Read the model definition and answer for the solid it produces. Units are mm, in the model's axes. Round coordinates to 2 decimals unless told otherwise and drop trailing zeros. Write each loop counter-clockwise with the first axis right and the second up, starting at its lowest first coordinate (ties: lowest second). Pieces come first, ordered by that corner, then holes. Notation, with made-up numbers: M 22.5,-20.5 L 53.5,-20.5 A23 ccw 53.5,4.5 Z; hole C 2.25,24 d7. An arc over 180 degrees is marked long. Use one line per item in the form item = value. Start each with the question number.
```python
from build123d import *

# Parameters (mm, degrees)
SKETCH_W  = 36
SKETCH_H  = 25
SKETCH_R  = 2
PAD_DEPTH = 11
FILLET_R  = 3


with BuildPart() as part:
    # Sketch → Pad (new body)
    with BuildSketch(Plane.XY):
        with Locations((0, 12.5)):
            Rectangle(SKETCH_W, SKETCH_H)
        with Locations((10, 16)):
            Circle(SKETCH_R, mode=Mode.SUBTRACT)
        with Locations((-10, 16)):
            Circle(SKETCH_R, mode=Mode.SUBTRACT)
    extrude(amount=PAD_DEPTH)

    # Fillet
    fillet_edges = [part.edges().sort_by_distance(p)[0] for p in [
        (-18, 25, 5.5),
        (18, 25, 5.5),
    ]]
    fillet(fillet_edges, radius=FILLET_R)


solid = part.part
```
Q1. Find section A-A on y = 16. Write down the section's boundary in (x, z).
Q2. For a pull along X with two mould halves and no side action, classify faces 1 (the face through (18, 11, 5)), 2 (the face through (0, 0, 5)), 3 (the face through (10, 18, 5)) as +X half, -X half, draft (parallel to the pull), parting line (faces both ways), or undercut.
Q3. Straight lines are drawn through the part: line 1 (X direction, y = 14.75, z = 10.75); line 2 (Y direction, x = -10, z = 6.25); line 3 (Y direction, x = -10.5, z = 4). For each, find the intervals that lie inside material, in ascending order. Write a range as [from, to].
Q4. Find section C-C on z = 4.75. Write down the section's boundary in (x, y), and give its area (3 significant figures).
Q5. Find section B-B on x = 10. Write down the section's boundary in (y, z).
Response:
q1.outline = M -18,0 L -12,0 L -12,11 L -18,11 Z; M -8,0 L 8,0 L 8,11 L -8,11 Z; M 12,0 L 18,0 L 18,11 L 12,11 Z
q2.face_1 = +X half
q2.face_2 = draft
q2.face_3 = undercut
q3.line_1 = [-18, -11.56], [-8.44, 8.44], [11.56, 18]
q3.line_2 = [0, 14], [18, 25]
q3.line_3 = [0, 14.06], [17.94, 25]
q4.outline = M -18,0 L 18,0 L 18,22 A3 ccw 15,25 L -15,25 A3 ccw -18,22 Z; hole C -10,16 d4; hole C 10,16 d4
q4.area = 871 mm²
q5.outline = M 0,0 L 14,0 L 14,11 L 0,11 Z; M 18,0 L 25,0 L 25,11 L 18,11 Z
